The listing builds one solid part. Answer for the finished solid, in the listing's coordinates (mm). Face numbers are marked on the shaded views. A direction names the side the tool comes from. Coordinates: 2 decimals unless noted, no trailing zeros. Order: outer loops, then holes, each group sorted by start corner. A loop starts at its lowest first (then second) coordinate and runs counter-clockwise, first axis right, second up.
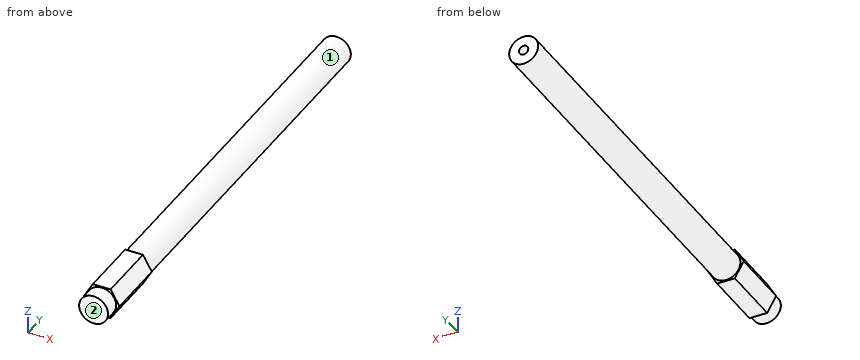
```python
from build123d import *

# Parameters (mm, degrees)
F0_R     = 4.7
F1_DEPTH = 150
F2_R     = 1.5
F3_DEPTH = 9.8
F6_DEPTH = 20


with BuildPart() as f1:
    # F0 (on Front) → F1 (new body)
    with BuildSketch(Plane.XZ):
        Circle(F0_R)
    extrude(amount=F1_DEPTH)

    # F2 (on face) → F3 (cut)
    with BuildSketch(Plane(origin=(0, 0, 0), x_dir=(-1, 0, 0), z_dir=(0, 1, 0))):
        Circle(F2_R)
    extrude(amount=-F3_DEPTH, mode=Mode.SUBTRACT)

    # F5 (on offset) → F6 (join)
    with BuildSketch(Plane.XZ.offset(145)):
        Polygon((2.887, 5.000431), (-2.887, 5.000431), (-5.774, 0), (-2.887, -5.000431), (2.887, -5.000431), (5.774, 0), align=None)
    extrude(amount=-F6_DEPTH)


solid = f1.part
```
(1) Find section D-D (y = -99.5). Write down the section's boundary in (x, z), and give its area (3 significant figures).
(2) For the marked faces 1 and 2, determine the directions among +Z, -Z, +X, -X, +Y, -Y from which every point of the face is accessible in a straight line to the end or side of a thin tool.
(3) Each of these flat-tipped pins is pushed along its axis until it touches: pin 1 Ø2 at (x, y) = (1, -15) entering from -Z; pin 2 Ø5 at (x, z) = (-0.5, 1.5) entering from +Y; pin 3 Ø4 at (x, y) = (1, -61) entering from +Z; pin 4 Ø1.5 at (y, z) = (-126, -3.5) entering from -X. Where does it stop, or does it pass through?
(4) Consider line 1 (Z direction, x = 0, y = -5.25); line 2 (Y direction, x = -3, z = 4.25); line 3 (Z direction, x = -3, y = -61). Determine where each line is inside the solid, lowest interval first.
(5) Find section B-B (y = -135.5). Write down the section's boundary in (x, z), and give its area (3 significant figures).
(6) Find section A-A (x = 0). Write down the section's boundary in (y, z).
(7) Find section C-C (z = -3.25). Write down the section's boundary in (x, y).
Findings below:
1. outline: circle Ø9.4 at (0, 0)
1. area: 69.4 mm2
2. face 1: +Y
2. face 2: +Z, -Z, +X, -X, -Y
3. pin 1: stops at z = -4.7
3. pin 2: stops at y = 0
3. pin 3: stops at z = 4.7
3. pin 4: stops at x = -4.19
4. line 1: z = -4.7 to -1.5, 1.5 to 4.7
4. line 2: y = -145 to -125
4. line 3: z = -3.62 to 3.62
5. outline: (-5.77, 0) - (-2.89, -5) - (2.89, -5) - (5.77, 0) - (2.89, 5) - (-2.89, 5) - close
5. area: 86.6 mm2
6. outline: (-150, -4.7) - (-145, -4.7) - (-145, -5) - (-125, -5) - (-125, -4.7) - (0, -4.7) - (0, -1.5) - (-9.8, -1.5) - (-9.8, 1.5) - (0, 1.5) - (0, 4.7) - (-125, 4.7) - (-125, 5) - (-145, 5) - (-145, 4.7) - (-150, 4.7) - close
7. outline: (-3.9, -145) - (-3.4, -145) - (-3.4, -150) - (3.4, -150) - (3.4, -145) - (3.9, -145) - (3.9, -125) - (3.4, -125) - (3.4, 0) - (-3.4, 0) - (-3.4, -125) - (-3.9, -125) - close
